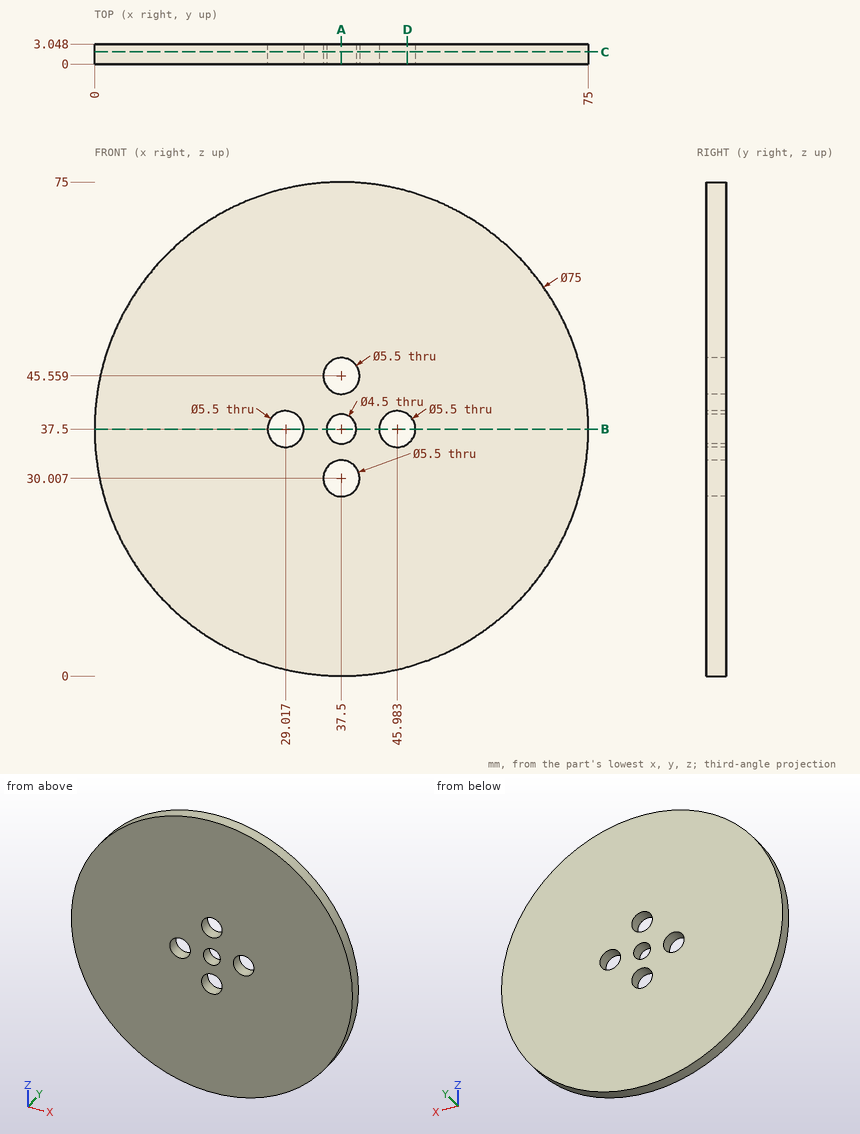
Print and shaded views of the part. All mm, measured from the part's lowest x, y and z. Coordinates: 2 decimals unless noted, no trailing zeros. Order: outer loops, then holes, each group sorted by start corner. A loop starts at its lowest first (then second) coordinate and runs counter-clockwise, first axis right, second up.
(1) Slice it at B-B, the plane z = 37.5. Write the cut outline in (x, y), and give its area (3 significant figures).
Check sheet entries:
outline: (0, 0) - (26.27, 0) - (26.27, 3.05) - (0, 3.05) - close; (31.77, 0) - (35.25, 0) - (35.25, 3.05) - (31.77, 3.05) - close; (39.75, 0) - (43.23, 0) - (43.23, 3.05) - (39.75, 3.05) - close; (48.73, 0) - (75, 0) - (75, 3.05) - (48.73, 3.05) - close
area: 181 mm2
(2) Slice it at C-C, the plane y = 1.85. Write the cut outline in (x, z), and give its area (3 significant figures).
Check sheet entries:
outline: circle Ø75 at (37.5, 37.5); hole circle Ø5.5 at (29.02, 37.5); hole circle Ø5.5 at (37.5, 30.01); hole circle Ø5.5 at (37.5, 45.56); hole circle Ø4.5 at (37.5, 37.5); hole circle Ø5.5 at (45.98, 37.5)
area: 4,310 mm2
(3) Probe L1, parallel to Z at x = 37.5, y = 2.1; L2, parallel to X at y = 0.7, z = 35 (1 decimal); L3, parallel to Z at x = 47, y = 2.3 (1 decimal). List the from-to ranges inside material, lowest first.
Check sheet entries:
L1: z = 0 to 27.26, 32.76 to 35.25, 39.75 to 42.81, 48.31 to 75
L2: x = 0.1 to 27.9, 30.2 to 44.8, 47.1 to 74.9
L3: z = 1.2 to 34.9, 40.1 to 73.8
(4) Slice it at D-D, the plane x = 47.5. Write the cut outline in (y, z), and give its area (3 significant figures).
Check sheet entries:
outline: (0, 1.36) - (3.05, 1.36) - (3.05, 35.21) - (0, 35.21) - close; (0, 39.79) - (3.05, 39.79) - (3.05, 73.64) - (0, 73.64) - close
area: 206 mm2
(5) Slice it at A-A, the plane x = 37.5. Write the cut outline in (y, z), and give its area (3 significant figures).
Check sheet entries:
outline: (0, 0) - (3.05, 0) - (3.05, 27.26) - (0, 27.26) - close; (0, 32.76) - (3.05, 32.76) - (3.05, 35.25) - (0, 35.25) - close; (0, 39.75) - (3.05, 39.75) - (3.05, 42.81) - (0, 42.81) - close; (0, 48.31) - (3.05, 48.31) - (3.05, 75) - (0, 75) - close
area: 181 mm2
(6) Pin check, flat tips, straight feed: pin 1 Ø1.5 at (y, z) = (2.5, 40) entering from -X; pin 2 Ø7 at (x, z) = (37.5, 45.56) entering from +Y. Stop position of each tip, or through.
Check sheet entries:
pin 1: stops at x = 0.04
pin 2: stops at y = 3.05
